The figure shows three views and two pictorial views of one solid part (mm, origin at its lowest corner). Answer the questions. A direction names the side the tool comes from. Round coordinates to 2 decimals unless told otherwise and drop trailing zeros. Order: outer loops, then holes, each group sorted by start corner. A loop starts at its lowest first (then second) coordinate and runs counter-clockwise, first axis right, second up. Notation, with made-up numbers: (10.5, 45) - (26.5, 45) arc R30 cw to (26.5, 84) - close; hole circle Ø1 at (23, -12). An arc over 180 degrees is marked (long way). Answer as a JSON object with one key per item and string values. Group by question number.
Q1. A cutting plane is placed at C-C on x = 1.75. Determine the outline of the cut face in (y, z).
Q2. The mould has two halves that part along X. Classify the marked faces 3, 4 and 5: pulls with the +X half, pulls with the -X half, needs draft (parallel to the pull), parting line crosses it, or undercut.
Q3. Consider line 1 (Y direction, x = 6.35, z = 43) (1 decimal); line 2 (X direction, y = 6.25, z = 9); line 3 (X direction, y = 7.5, z = 48) (1 decimal). Determine where each line is inside the solid, lowest interval first.
Q4. A cutting plane is placed at B-B on z = 21. Determine the outline of the cut face in (x, y).
Q5. Given pin 1 Ø4 at (x, z) = (8, 27.5) entering from +Y; pin 2 Ø4 at (y, z) = (9.5, 46) entering from -X (3 decimals); pin 3 Ø1.5 at (x, z) = (3.5, 6) entering from -Y, each flat-ended and moving along its own axis, determine where each tip first touches the part or whether it passes through.
Q6. A tool of negligible diameter and unlimited length cuts with its end or side. For the marked faces 1 and 2, from which of +Z, -Z, +X, -X, +Y, -Y can it reach the whole face along a straight path? Write none if from no direction.
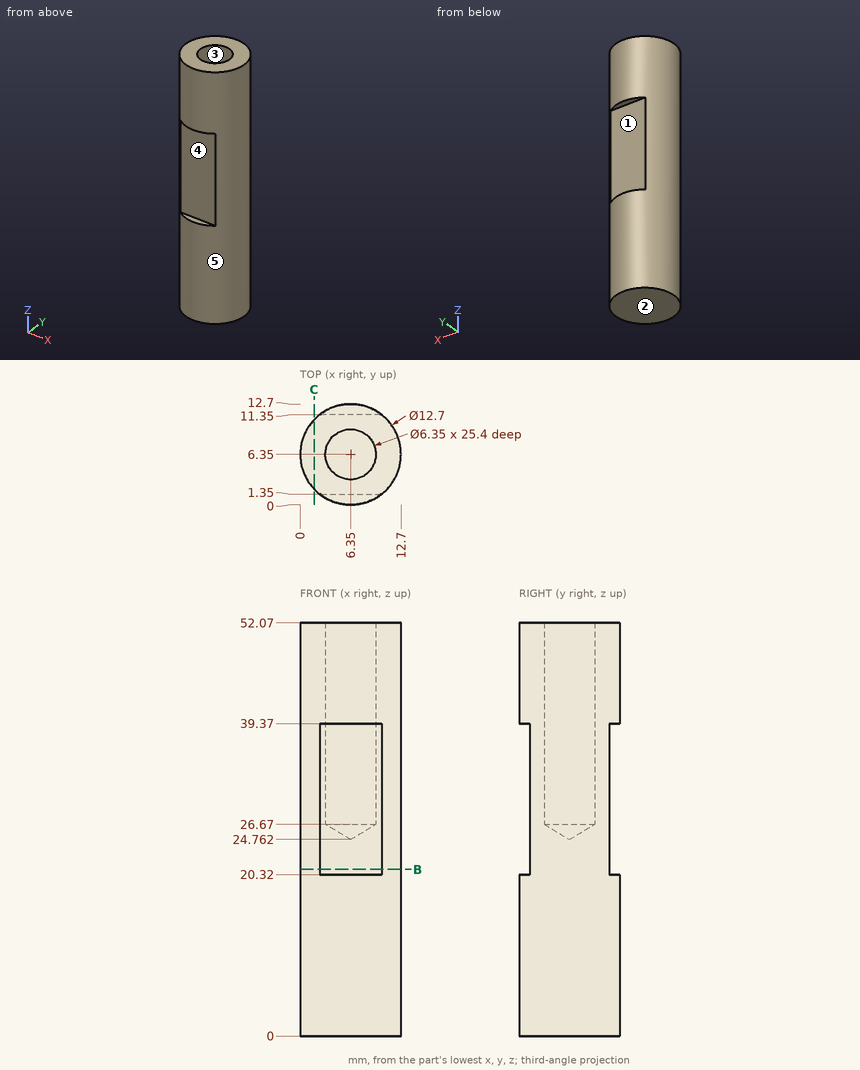
Result set:
{
 "1": {"outline": "(1.97, 0) - (10.73, 0) - (10.73, 52.07) - (1.97, 52.07) - close"},
 "2": {"face 3": "undercut", "face 4": "needs draft", "face 5": "parting line crosses it"},
 "3": {"line 1": "y = 0 to 3.2, 9.5 to 12.7", "line 2": "x = 0 to 12.7", "line 3": "x = 0.1 to 3.4, 9.3 to 12.6"},
 "4": {"outline": "(2.44, 1.35) - (10.26, 1.35) arc R6.35 ccw to (10.26, 11.35) - (2.44, 11.35) arc R6.35 ccw to start"},
 "5": {"pin 1": "stops at y = 11.35", "pin 2": "stops at x = 0.105", "pin 3": "stops at y = 0.36"},
 "6": {"face 1": "+X, -X, +Y", "face 2": "-Z, +X, -X, +Y, -Y"}
}
